For this review, take the finished solid that the model builds, in its own axes (mm). A direction names the side the tool comes from. Give positions to 0.01 mm unless a question says otherwise; leave off trailing zeros. Write each loop counter-clockwise with the first axis right and the second up, starting at its lowest first coordinate (ties: lowest second). Pieces come first, ordered by that corner, then holes.
Q1. We need section B-B (z = -87). Write out the cut boundary in (x, y) (3 decimals).
Q2. We need section D-D (z = 91). Write out the cut boundary in (x, y).
Q3. Mouldability with a two-part tool opening along X and no side actions: class faces 1 (the flat face through (97.594, 157.324, 2.87)), 2 (the flat face through (-135, 3, 3)), 3 (the flat face through (125, 2, 3)), 4 (the flat face through (-1, 193.35, 3)) as released by +X, released by -X, zero draft, split by the parting line, or undercut.
Q4. We need section C-C (y = -46). Write out the cut boundary in (x, z), then the cut area to 3 significant figures.
Q5. For line 1 (X direction, y = 20, z = 116.5); line 2 (Y direction, x = -18, z = -131.5); line 3 (Y direction, x = -116.5, z = -141), list the stretches that pass through material, from the lowest coordinate up.
Q6. Insertion check: P1, Ø8, axis at x = -35.5, z = 149, coming from the +Y side; P2, Ø9, axis at y = 221.5, z = -98, coming from the -X side (3 decimals); P3, Ø24, axis at x = 10.5, y = 223.5, coming from the +Z side. Each pin has a flat end and moves straight along its axis. Give the tip position at first contact, or say it passes through.
Q7. Machinability: for faces 5 (the flat face through (34.975, 213, -95)), 6 (the flat face through (-1, 218, -65)), 7 (the flat face through (-125, -2, 3)), 8 (the flat face through (-1, 218, -125)), which of the approach directions +Z, -Z, +X, -X, +Y, -Y give a long, thin tool a straight path to every point of the face, cutting with its end or side? Answer none if there is none.
Q8. We need section A-A (x = 11). Write out the cut boundary in (y, z), then the cut area to 3 significant figures.
```python
from build123d import *

# Parameters (mm, degrees)
BOSS_EXTRUDE1_DEPTH = 205
SKETCH2_W           = 69.949988916
SKETCH2_H           = 40
CUT_EXTRUDE1_DEPTH  = 204.35
BOSS_EXTRUDE2_START = 203.35
SKETCH3_W           = 89.949988916
SKETCH3_H           = 60
SKETCH3_W_2         = 69.949988916
SKETCH3_H_2         = 40
BOSS_EXTRUDE2_DEPTH = 30


with BuildPart() as part:
    # Sketch1 → Boss-Extrude1 (new body, symmetric)
    with BuildSketch(Plane.XY):
        Polygon((-125, 108.94), (-54.45, 193.35), (54.45, 193.35), (125, 108.94), (125, -108.94), (135, -108.94), (135, 112.568729132), (59.1248826, 203.35), (-59.1248826, 203.35), (-135, 112.568729132), (-135, -108.94), (-125, -108.94), align=None)
    extrude(amount=BOSS_EXTRUDE1_DEPTH, both=True)

    # Sketch2 → Cut-Extrude1 (cut, through all)
    with BuildSketch(Plane(origin=(0, 0, 0), x_dir=(1, 0, 0), z_dir=(0, 1, 0))):
        with Locations((0, 95)):
            Rectangle(SKETCH2_W, SKETCH2_H)
    extrude(amount=CUT_EXTRUDE1_DEPTH, mode=Mode.SUBTRACT)

    # Sketch3 → Boss-Extrude2 (add)
    with BuildSketch(Plane(origin=(0, 0, 0), x_dir=(1, 0, 0), z_dir=(0, 1, 0)).offset(BOSS_EXTRUDE2_START)):
        with Locations((0, 95)):
            Rectangle(SKETCH3_W, SKETCH3_H)
        with Locations((0, 95)):
            Rectangle(SKETCH3_W_2, SKETCH3_H_2, mode=Mode.SUBTRACT)
    extrude(amount=BOSS_EXTRUDE2_DEPTH)


solid = part.part
```
Computed:
1. outline: (-135, -108.94) - (-125, -108.94) - (-125, 108.94) - (-54.45, 193.35) - (-34.975, 193.35) - (-34.975, 233.35) - (-44.975, 233.35) - (-44.975, 203.35) - (-59.125, 203.35) - (-135, 112.569) - close; (34.975, 193.35) - (54.45, 193.35) - (125, 108.94) - (125, -108.94) - (135, -108.94) - (135, 112.569) - (59.125, 203.35) - (44.975, 203.35) - (44.975, 233.35) - (34.975, 233.35) - close
2. outline: (-135, -108.94) - (-125, -108.94) - (-125, 108.94) - (-54.45, 193.35) - (54.45, 193.35) - (125, 108.94) - (125, -108.94) - (135, -108.94) - (135, 112.57) - (59.12, 203.35) - (-59.12, 203.35) - (-135, 112.57) - close
3. face 1: released by +X
3. face 2: released by -X
3. face 3: undercut
3. face 4: undercut
4. outline: (-135, -205) - (-125, -205) - (-125, 205) - (-135, 205) - close; (125, -205) - (135, -205) - (135, 205) - (125, 205) - close
4. area: 8,200 mm2
5. line 1: x = -135 to -125, 125 to 135
5. line 2: y = 193.35 to 203.35
5. line 3: y = 119.11 to 134.7
6. P1: stops at y = 203.35
6. P2: stops at x = -44.975
6. P3: stops at z = -65
7. face 5: +Y, -Y
7. face 6: +Z, +X, -X, +Y
7. face 7: +Z, -Z, -Y
7. face 8: -Z, +X, -X, +Y
8. outline: (193.35, -205) - (203.35, -205) - (203.35, -125) - (233.35, -125) - (233.35, -115) - (193.35, -115) - close; (193.35, -75) - (233.35, -75) - (233.35, -65) - (203.35, -65) - (203.35, 205) - (193.35, 205) - close
8. area: 4,300 mm2
